Model file for the job. Use its own axes, mm. A direction names the side the tool comes from. Give positions to 0.01 mm unless a question says otherwise; leave off trailing zeros. Loops run counter-clockwise (first coordinate to the right, second up) from the corner with the lowest first, then second, coordinate; pieces in that order, holes last. Notation, with made-up numbers: M -40,8 L 8,8 A14 ccw 8,25 Z; hole C 75,16 d1. An arc over 180 degrees is marked long. Answer in a Markdown table with one row per item.
Solid Edge part; units mm, degrees
sketch "Sketch1" plane through (0, 0, 0) normal (0, -1, 0) x (1, 0, 0)
  circle A0 centre (0, 0) radius 4
extrude "Protrusion1" add sketch "Sketch1" against normal blind 25
sketch "Sketch2" plane through (0, 0, 0) normal (0, -1, 0) x (1, 0, 0)
  circle A0 centre (0, 0) radius 6.5
extrude "Protrusion2" add sketch "Sketch2" along normal blind 8
sketch "Sketch3" plane through (0, -8, 0) normal (0, -1, 0) x (1, 0, 0)
  line L0 (-1.7321, -3) -> (1.7321, -3)
  line L1 (1.7321, -3) -> (3.4641, 0)
  line L2 (3.4641, 0) -> (1.7321, 3)
  line L3 (1.7321, 3) -> (-1.7321, 3)
  line L4 (-1.7321, 3) -> (-3.4641, 0)
  line L5 (-3.4641, 0) -> (-1.7321, -3)
extrude "Cutout1" cut sketch "Sketch3" against normal blind 5
fillet "Round1" radius 0.5 1 edges at (-6.5, -8, 0)
chamfer "Chamfer1" distance 0.625 angle 45 1 edges at (-4, 25, 0)
chamfer "Chamfer2" distance 0.2 angle 45 6 edges at (0, -8, 3) (-2.5981, -8, 1.5) (-2.5981, -8, -1.5) (0, -8, -3) (2.5981, -8, -1.5) (2.5981, -8, 1.5)
cosmetic_thread "Thread1"
properties part number "16" material "Stainless steel"
Q1. 3-axis set-ups, long thin cutter, end or side, ignore diameter. For faces 1 (the face through (2.6, -5.4, 1.5)), 2 (the face through (-3, -8, -3)), 3 (the face through (3, 0, -3)): which of +Z, -Z, +X, -X, +Y, -Y reach the whole face in a straight line?
Reported:
| item | result |
|---|---|
| face 1 | -Y |
| face 2 | +Z, -Z, +X, -X, -Y |
| face 3 | +Y |
Q2. Saw through at B-B (y = 18.5). Give the cut face in (x, z).
Reported:
| item | result |
|---|---|
| outline | C 0,0 d8 |
Q3. Drop flat-ended pins along their axis: pin 1 (3 mm diameter, centred on y = 2, z = -5, fed in from -X); pin 2 (2 mm diameter, centred on y = 16.5, z = -2, fed in from +X); pin 3 (2 mm diameter, centred on x = 2.5, y = 0.5, fed in from +Z). Give the stop position or say it passes through.
Reported:
| item | result |
|---|---|
| pin 1 | x = -1.94 |
| pin 2 | x = 3.87 |
| pin 3 | z = 6.29 |
Q4. Probe probe 1 along Y at (x, z) = (-2.25, -0.75); probe 2 along Y at (x, z) = (-2.25, -5.5); probe 3 along X at (y, z) = (-5, 1.75). List the from-to ranges inside material, lowest first.
Reported:
| item | result |
|---|---|
| probe 1 | -3 to 25 |
| probe 2 | -8 to 0 |
| probe 3 | -6.26 to -2.45, 2.45 to 6.26 |
Q5. Mould opens along Z. For faces 4 (the face through (0, 25, 0)), 5 (the face through (0, -5, 3)), 6 (the face through (-0.867, 12.017, -3.905)) say: released by +Z, released by -Z, zero draft, split by the parting line, or undercut.
Reported:
| item | result |
|---|---|
| face 4 | zero draft |
| face 5 | undercut |
| face 6 | split by the parting line |
Q6. Saw through at A-A (x = 0). Give the cut face in (y, z) (3 decimals), and give its area (3 significant figures).
Reported:
| item | result |
|---|---|
| outline | M -8,-6 A0.5 ccw -7.5,-6.5 L 0,-6.5 L 0,-4 L 24.375,-4 L 25,-3.375 L 25,3.375 L 24.375,4 L 0,4 L 0,6.5 L -7.5,6.5 A0.5 ccw -8,6 L -8,3.2 L -7.8,3 L -3,3 L -3,-3 L -7.8,-3 L -8,-3.2 Z |
| area | 273 mm² |
